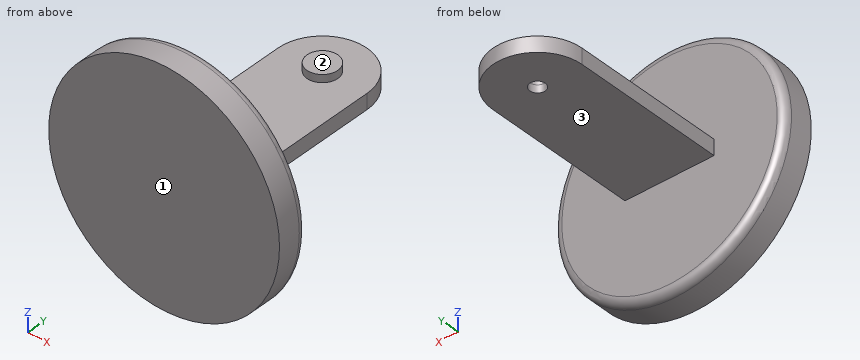
```python
from build123d import *

# Parameters (mm, degrees)
SKETCH1_R                = 75
BOSS_EXTRUDE1_DEPTH      = 20
FILLET1_R                = 5
BOSS_EXTRUDE2_DEPTH      = 5
BOSS_EXTRUDE2_DEPTH_BACK = 5
SKETCH3_R                = 10
BOSS_EXTRUDE4_DEPTH      = 10
SKETCH4_R                = 5
CUT_EXTRUDE2_DEPTH       = 5
CUT_EXTRUDE2_DEPTH_BACK  = 5


with BuildPart() as part:
    # Sketch1 → Boss-Extrude1 (new body)
    with BuildSketch(Plane(origin=(0, 0, 0), x_dir=(1, 0, 0), z_dir=(0, 1, 0))):
        Circle(SKETCH1_R)
    extrude(amount=BOSS_EXTRUDE1_DEPTH)

    # Fillet1
    fillet1_edges = [part.edges().sort_by_distance(p)[0] for p in [
        (-75, 20, 0),
    ]]
    fillet(fillet1_edges, radius=FILLET1_R)

    # Sketch2 → Boss-Extrude2 (add, two sides)
    with BuildSketch(Plane.XY) as boss_extrude2_sk:
        with BuildLine():
            Line((-28.958565119, 120), (-28.958565119, 20))
            Line((-28.958565119, 20), (28.958565119, 20))
            Line((28.958565119, 20), (28.958565119, 120))
            ThreePointArc((28.958565119, 120), (0, 148.958565119), (-28.958565119, 120))
        make_face()
    extrude(amount=BOSS_EXTRUDE2_DEPTH)
    extrude(boss_extrude2_sk.sketch, amount=-BOSS_EXTRUDE2_DEPTH_BACK)

    # Sketch3 → Boss-Extrude4 (add)
    with BuildSketch(Plane.XY):
        with Locations((0, 120)):
            Circle(SKETCH3_R)
    extrude(amount=BOSS_EXTRUDE4_DEPTH)

    # Sketch4 → Cut-Extrude2 (cut, two sides)
    with BuildSketch(Plane.XY) as cut_extrude2_sk:
        with Locations((0, 120)):
            Circle(SKETCH4_R)
    extrude(amount=CUT_EXTRUDE2_DEPTH, mode=Mode.SUBTRACT)
    extrude(cut_extrude2_sk.sketch, amount=-CUT_EXTRUDE2_DEPTH_BACK, mode=Mode.SUBTRACT)


solid = part.part
```
For this review, take the finished solid that the model builds, in its own axes (mm). Face numbers are marked on the shaded views. A direction names the side the tool comes from. Round coordinates to 2 decimals unless told otherwise and drop trailing zeros. Write each loop counter-clockwise with the first axis right and the second up, starting at its lowest first coordinate (ties: lowest second). Pieces come first, ordered by that corner, then holes. Notation, with made-up numbers: (19.25, 26) - (40.25, 26) arc R16 cw to (40.25, 43) - close; hole circle Ø9 at (73.25, 45.25). An arc over 180 degrees is marked (long way). Write each question's results on one line, items separated by ' | '.
Item 1: Take a section at B-B on y = 43. State the section outline as (x, z) points.
Calculated:
outline: (-28.96, -5) - (28.96, -5) - (28.96, 5) - (-28.96, 5) - close
Item 2: For the marked faces 1, 2 and 3, list the 3-axis set-ups (+Z, -Z, +X, -X, +Y, -Y) from which the entire face can be reached by the end or side of a thin tool; tool diameter is ignored.
Calculated:
face 1: +Z, -Z, +X, -X, -Y | face 2: +Z, +X, -X, +Y | face 3: -Z, +X, -X, +Y
Item 3: For pin 1 (4 mm diameter, centred on x = 6.5, y = 93, fed in from +Z); pin 2 (3 mm diameter, centred on y = 75, z = 1, fed in from -X); pin 3 (16 mm diameter, centred on x = 0, y = 120, fed in from +Z), all flat-tipped, find the tip position at first contact; note any pin that passes through.
Calculated:
pin 1: stops at z = 5 | pin 2: stops at x = -28.96 | pin 3: stops at z = 10
Item 4: Take a section at A-A on x = 0. State the section outline as (y, z) points.
Calculated:
outline: (0, -75) - (15, -75) arc R5 ccw to (20, -70) - (20, -5) - (115, -5) - (115, 5) - (125, 5) - (125, -5) - (148.96, -5) - (148.96, 5) - (130, 5) - (130, 10) - (110, 10) - (110, 5) - (20, 5) - (20, 70) arc R5 ccw to (15, 75) - (0, 75) - close
Item 5: To check wall thickness, follow line 1 along Y through (x, z) = (0, -3.6); line 2 along Z through (x, y) = (-7, 33.5); line 3 along Y through (x, z) = (-17, 59.5). State the ranges of each line that lie inside material, in increasing order. Write a range as from..to.
Calculated:
line 1: y = 0..115, 125..148.96 | line 2: z = -5..5 | line 3: y = 0..20
